Read the model definition and answer for the solid it produces. Units are mm, in the model's axes. A direction names the side the tool comes from. Round coordinates to 2 decimals unless told otherwise and drop trailing zeros. Order: outer loops, then holes, each group sorted by start corner. A loop starts at its lowest first (then second) coordinate and runs counter-clockwise, first axis right, second up. Notation, with made-up numbers: (37, 33.25) -> (89, 33.25) arc R24 ccw to (89, 51.25) -> close; hole circle Ø7 at (14, 2). An arc over 180 degrees is marked (long way). Answer as a JSON object with one key per item and string values. Group by question number.
Item 1: Section B-B, the plane x = 11 is taken. Write down the section's boundary in (y, z), plus the area to 3 significant figures.
Item 2: Section C-C, the plane y = 8.5 is taken. Write down the section's boundary in (x, z), plus the area to 3 significant figures.
Item 3: For faces 4 (the flat face through (14, 0, 6)), 5 (the flat face through (11, 3, -4.55)), 6 (the flat face through (22.231, 19.936, 2.958)), determine the directions among +Z, -Z, +X, -X, +Y, -Y from which every point of the face is accessible in a straight line to the end or side of a thin tool.
Item 4: Section A-A, the plane y = 5 is taken. Write down the section's boundary in (x, z), plus the area to 3 significant figures.
Item 5: Given P1, Ø3, axis at y = 21.5, z = -2, coming from the -X side; P2, Ø4.5, axis at x = 9, z = -1.5, coming from the -Y side; P3, Ø8, axis at y = 24.5, z = -2.5, coming from the -X side, each flat-ended and moving along its own axis, determine where each tip first touches the part or whether it passes through.
Item 6: Consider probe 1 along Z at (x, y) = (4.5, 5); probe 2 along Y at (x, z) = (5, -3.25); probe 3 along Z at (x, y) = (25.5, 10.5). Determine where each line is inside the solid, lowest interval first. Write a range as from..to.
Item 7: Section D-D, the plane z = -2 is taken. Write down the section's boundary in (x, y), plus the area to 3 significant figures.
Item 8: The mould has two halves that part along Z. Classify faces 1 (the flat face through (-9.393, 16.269, 0.098)), 2 (the flat face through (22.377, 19.936, -3.042)), 3 (the flat face through (10, 17, 7)): pulls with the +Z half, pulls with the -Z half, needs draft (parallel to the pull), parting line crosses it, or undercut.
from build123d import *

# Parameters (mm, degrees)
EXTRUDE003_DEPTH = 33
SKETCH001_W      = 34.669946
SKETCH001_H      = 5.9
EXTRUDE001_DEPTH = 4.55
EXTRUDE_DEPTH    = 7


with BuildPart() as extrude003:
    # Sketch002 (on Cut) → Extrude003 (new body)
    with BuildSketch(Plane.XZ):
        Polygon((27.5, 6), (27.5, -6), (17.107695, 0), align=None)
    extrude(amount=-EXTRUDE003_DEPTH)


with BuildPart() as extrude001:
    # Sketch001 (on Extrude) → Extrude001 (new body, symmetric)
    with BuildSketch(Plane.XY):
        with Locations((12.538995, 2.95)):
            Rectangle(SKETCH001_W, SKETCH001_H)
    extrude(amount=EXTRUDE001_DEPTH, both=True)


with BuildPart() as cut001:
    # Sketch → Extrude (new body, symmetric)
    with BuildSketch(Plane.XY):
        Polygon((0, 0), (-19.052559, 33), (27.5, 33), (27.5, 0), align=None)
    extrude(amount=EXTRUDE_DEPTH, both=True)

    # Cut: cut Extrude001
    add(extrude001.part, mode=Mode.SUBTRACT)

    # Cut001: cut Extrude003
    add(extrude003.part, mode=Mode.SUBTRACT)


solid = cut001.part
Values found:
{
 "1": {"outline": "(0, -7) -> (33, -7) -> (33, 7) -> (0, 7) -> (0, 4.55) -> (5.9, 4.55) -> (5.9, -4.55) -> (0, -4.55) -> close", "area": "408 mm2"},
 "2": {"outline": "(-4.91, -7) -> (27.5, -7) -> (27.5, -6) -> (17.11, 0) -> (27.5, 6) -> (27.5, 7) -> (-4.91, 7) -> close", "area": "391 mm2"},
 "3": {"face 4": "+Z, -Z, +X, -X, -Y", "face 5": "+X, -X, -Y", "face 6": "+X, +Y, -Y"},
 "4": {"outline": "(-2.89, -7) -> (27.5, -7) -> (27.5, -6) -> (24.99, -4.55) -> (-2.89, -4.55) -> close; (-2.89, 4.55) -> (24.99, 4.55) -> (27.5, 6) -> (27.5, 7) -> (-2.89, 7) -> close", "area": "145 mm2"},
 "5": {"P1": "x = -13.28", "P2": "y = 5.9", "P3": "x = -16.45"},
 "6": {"probe 1": "-7..-4.55, 4.55..7", "probe 2": "5.9..33", "probe 3": "-7..-4.85, 4.85..7"},
 "7": {"outline": "(-19.05, 33) -> (-3.41, 5.9) -> (20.57, 5.9) -> (20.57, 33) -> close", "area": "862 mm2"},
 "8": {"face 1": "needs draft", "face 2": "undercut", "face 3": "pulls with the +Z half"}
}
